Here's how the part is built. I have some questions about the finished solid (model axes, mm). Coordinates: 2 decimals unless noted, no trailing zeros. Write each loop counter-clockwise with the first axis right and the second up, starting at its lowest first coordinate (ties: lowest second). Pieces come first, ordered by that corner, then holes. Notation, with made-up numbers: (-33.75, 50) -> (7.25, 50) arc R21 cw to (7.25, 70) -> close; hole circle Ø8 at (50.5, 6). An arc over 180 degrees is marked (long way). Use a Markdown table: item, result. Add a question column.
Item 1: If I drill on line 1 along X through (y, z) = (12.25, 80); line 2 along Z through (x, y) = (0, 9.25); line 3 along X through (y, z) = (13.25, 64), over which ranges is the centre line in solid material (lowest first)? Write a range as from..to.
Item 2: Imagine slicing it at A-A, the plane x = 0. Write out the boundary of the cut face in (y, z).
Item 3: Imagine slicing it at B-B, the plane z = 80. Write out the boundary of the cut face in (x, y), and give its area (3 significant figures).
Item 4: Imagine slicing it at C-C, the plane y = 6.25. Write out the boundary of the cut face in (x, z), and give its area (3 significant figures).
```python
from build123d import *

# Parameters (mm, degrees)
SKETCH1_W           = 500
SKETCH1_H           = 760
BOSS_EXTRUDE1_DEPTH = 20
CUT_EXTRUDE2_REACH  = 22
SKETCH3_R           = 125


with BuildPart() as part:
    # Sketch1 → Boss-Extrude1 (new body)
    with BuildSketch(Plane(origin=(0, 0, 0), x_dir=(1, 0, 0), z_dir=(0, 1, 0))):
        Rectangle(SKETCH1_W, SKETCH1_H)
    extrude(amount=BOSS_EXTRUDE1_DEPTH)

    # Sketch3 → Cut-Extrude2 (cut, up to next)
    with BuildSketch(Plane(origin=(0, 20, 0), x_dir=(1, 0, 0), z_dir=(0, 1, 0)), mode=Mode.PRIVATE) as cut_extrude2_sk1:
        with Locations((0, -80)):
            Circle(SKETCH3_R)
    cut_extrude2_tool1 = extrude(cut_extrude2_sk1.sketch, amount=-CUT_EXTRUDE2_REACH, mode=Mode.PRIVATE) & part.part
    add(cut_extrude2_tool1.solids().sort_by_distance((0, 20, 80))[0], mode=Mode.SUBTRACT)


solid = part.part
```
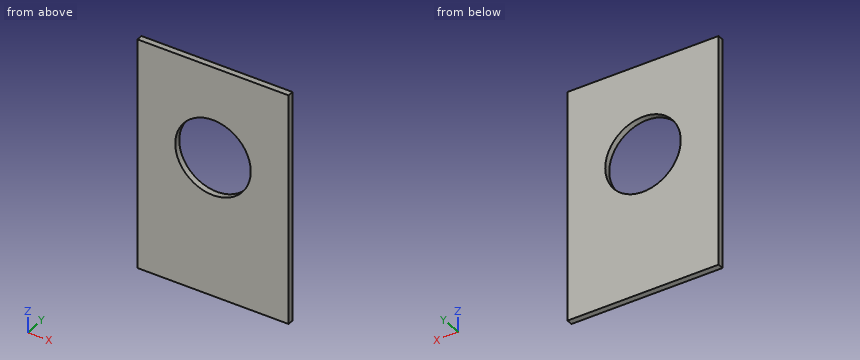
Ans:
| question | item | result |
|---|---|---|
| 1 | line 1 | x = -250..-125, 125..250 |
| 1 | line 2 | z = -380..-45, 205..380 |
| 1 | line 3 | x = -250..-123.97, 123.97..250 |
| 2 | outline | (0, -380) -> (20, -380) -> (20, -45) -> (0, -45) -> close; (0, 205) -> (20, 205) -> (20, 380) -> (0, 380) -> close |
| 3 | outline | (-250, 0) -> (-125, 0) -> (-125, 20) -> (-250, 20) -> close; (125, 0) -> (250, 0) -> (250, 20) -> (125, 20) -> close |
| 3 | area | 5,000 mm^2 |
| 4 | outline | (-250, -380) -> (250, -380) -> (250, 380) -> (-250, 380) -> close; hole circle Ø250 at (0, 80) |
| 4 | area | 331,000 mm^2 |
